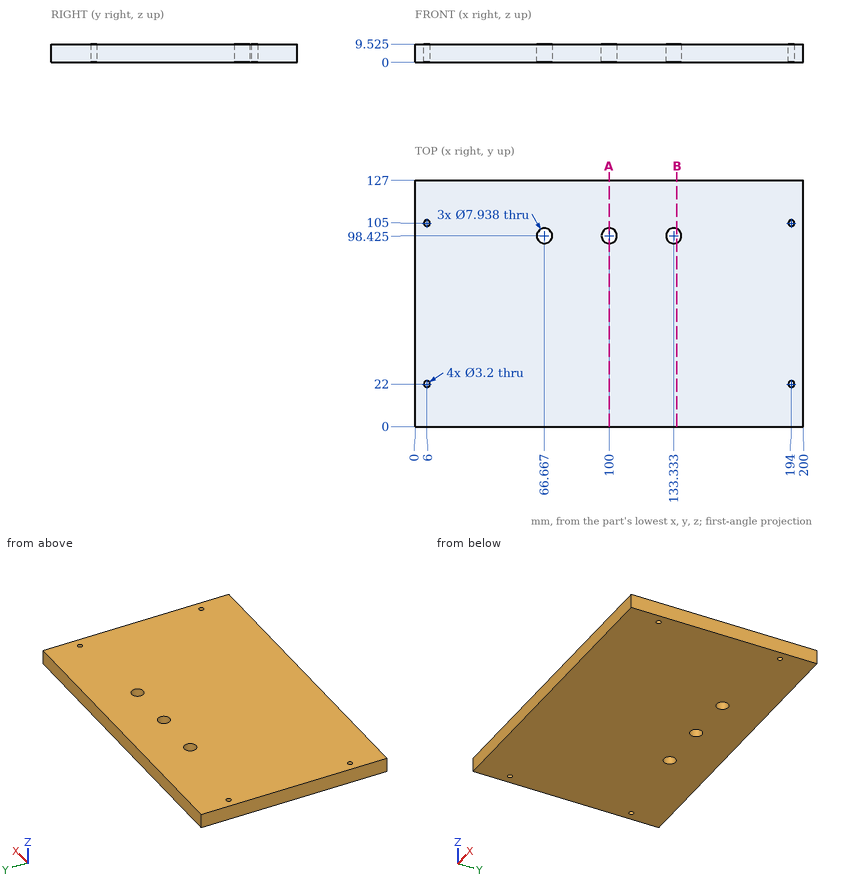
Geometry check sheet. Reference: drawing and pictorial views, mm from the part's lowest x, y, z. Round coordinates to 2 decimals unless told otherwise and drop trailing zeros. Loops run counter-clockwise (first coordinate to the right, second up) from the corner with the lowest first, then second, coordinate; pieces in that order, holes last. Notation, with made-up numbers: (33, -30.75) - (87, -30.75) arc R17 cw to (87, -25.75) - close; hole circle Ø8 at (83, 34). An arc over 180 degrees is marked (long way). Write item = value, one per line. Start each with the question number.
Q1. Depth check by flat-ended pin: P1, Ø10.5, axis at x = 133.33, y = 98.42, coming from the -Z side; P2, Ø2.5, axis at x = 194, y = 22, coming from the -Z side. Enter the tip coordinate at first touch or a pass-through.
Q2. Section check A-A (x = 100). Record the boundary of the cut face in (y, z) (1 decimal).
Q3. Section check B-B (x = 135). Record the boundary of the cut face in (y, z) (1 decimal).
Q4. Thickness scan on L1, parallel to X at y = 22, z = 5; L2, parallel to X at y = 102, z = 3.75 (1 decimal). Record the ranges inside material, lowest first.
Derived:
q1.P1 = 0
q1.P2 = through
q2.outline = (0, 0) - (94.5, 0) - (94.5, 9.5) - (0, 9.5) - close; (102.4, 0) - (127, 0) - (127, 9.5) - (102.4, 9.5) - close
q3.outline = (0, 0) - (94.8, 0) - (94.8, 9.5) - (0, 9.5) - close; (102, 0) - (127, 0) - (127, 9.5) - (102, 9.5) - close
q4.L1 = 0 to 4.4, 7.6 to 192.4, 195.6 to 200
q4.L2 = 0 to 64.9, 68.4 to 98.3, 101.7 to 131.6, 135.1 to 200
